Work out the finished part from the listing and answer in its coordinate system (mm). A direction names the side the tool comes from. Give positions to 0.01 mm unless a question says otherwise; leave off trailing zeros. Write each loop counter-clockwise with the first axis right and the second up, starting at its lowest first coordinate (ties: lowest second). Pieces come first, ordered by that corner, then holes. Notation, with made-up numbers: (51, -3) -> (98, -3) arc R32 cw to (98, 26) -> close; hole circle Ø1 at (22, -38). An arc over 180 degrees is marked (long way). Use a Markdown table: item, result. Add a question column.
Q1. Section B-B, the plane z = 45 is taken. Give the vertices of the cut face in (x, y).
Q2. Section A-A, the plane y = -6 is taken. Give the vertices of the cut face in (x, z).
Q3. Section C-C, the plane x = -17 is taken. Give the vertices of the cut face in (y, z).
Q4. For faces 1 (the face through (0, -7, 65)), 2 (the face through (-1, -14, 0.5)), 3 (the face through (3.3, -2.53, -1.23)), determine the directions among +Z, -Z, +X, -X, +Y, -Y from which every point of the face is accessible in a straight line to the end or side of a thin tool.
Q5. Each of these flat-tipped pins is pushed along its axis until it touches: pin 1 Ø3 at (y, z) = (-11, 14.5) entering from +X; pin 2 Ø3 at (x, y) = (9.5, 5.5) entering from -Z; pin 3 Ø4 at (x, z) = (-18, 30) entering from -Y. Where does it stop, or does it pass through?
Q6. Section D-D, the plane y = 6.5 is taken. Give the vertices of the cut face in (x, z).
Q7. Consider line 1 (Z direction, x = 14.5, y = 13.5); line 2 (Y direction, x = 0, z = 66.4); line 3 (X direction, y = 5.5, z = 54.5). Determine where each line is inside the solid, lowest interval first.
Q8. For a pull along Z with two mould halves and no side action, classify faces 4 (the face through (7.31, 12.62, 55.27)), 5 (the face through (-31.096, 0.559, 32.99)), 6 (the face through (6.68, 12.64, 11.65)), 7 (the face through (0, 0, 2.5)) as pulls with the +Z half, pulls with the -Z half, needs draft (parallel to the pull), parting line crosses it, or undercut.
from build123d import *

# Parameters (mm, degrees)
SKETCH_1_R          = 9.1
EXTRUDE_1_DEPTH     = 65
EXTRUDE_2_DEPTH     = 2.5
EXTRUDE_3_DEPTH     = 2.5
SKETCH_7_W          = 30
SKETCH_7_H          = 64
CUT_EXTRUDE_4_DEPTH = 4.5
SKETCH_8_W          = 30
SKETCH_8_H          = 64
CUT_EXTRUDE_5_DEPTH = 4.5
SKETCH_4_R          = 4.159545235
SKETCH_4_R_2        = 2.25
EXTRUDE_4_DEPTH     = 2.5
SKETCH_10_R         = 2.25
CUT_EXTRUDE_6_DEPTH = 2.5
SKETCH_11_R         = 4.25
SKETCH_11_R_2       = 2.25
EXTRUDE_5_DEPTH     = 4.5
SKETCH_3_R          = 4.25
SKETCH_3_R_2        = 2.25
EXTRUDE_6_DEPTH     = 2.5


with BuildPart() as part:
    # Эскиз1 → Бобышка-Вытянуть1 (new body)
    with BuildSketch(Plane.XY):
        with BuildLine():
            Line((-15.348477888, 15.359663741), (14.645527362, 14.759956259))
            ThreePointArc((14.645527362, 14.759956259), (29.785323334, -0.997609119), (14.027757956, -16.137405091))
            Line((14.027757956, -16.137405091), (-15.966247294, -15.537697609))
            ThreePointArc((-15.966247294, -15.537697609), (-31.106043266, 0.219867769), (-15.348477888, 15.359663741))
        make_face()
        with Locations((-15.657362591, -0.089016934)):
            Circle(SKETCH_1_R, mode=Mode.SUBTRACT)
        with Locations((14.336642659, -0.688724416)):
            Circle(SKETCH_1_R, mode=Mode.SUBTRACT)
    extrude(amount=EXTRUDE_1_DEPTH)

    # Эскиз2 → Бобышка-Вытянуть2 (add)
    with BuildSketch(Plane.XY.offset(65)):
        with BuildLine():
            Line((-15.966247294, -15.537697609), (14.027757956, -16.137405091))
            ThreePointArc((14.027757956, -16.137405091), (29.785323334, -0.997609119), (14.645527362, 14.759956259))
            Line((14.645527362, 14.759956259), (-15.348477888, 15.359663741))
            ThreePointArc((-15.348477888, 15.359663741), (-31.106043266, 0.219867769), (-15.966247294, -15.537697609))
        make_face()
        with BuildLine():
            Line((-15.378463262, 13.859963479), (14.615541988, 13.260255996))
            ThreePointArc((14.615541988, 13.260255996), (28.285623072, -0.967623745), (14.05774333, -14.637704829))
            Line((14.05774333, -14.637704829), (-15.93626192, -14.037997346))
            ThreePointArc((-15.93626192, -14.037997346), (-29.606343003, 0.189882395), (-15.378463262, 13.859963479))
        make_face(mode=Mode.SUBTRACT)
    extrude(amount=EXTRUDE_2_DEPTH)

    # Эскиз5 → Бобышка-Вытянуть3 (add)
    with BuildSketch(Plane(origin=(0, 0, 0), x_dir=(-1, 0, 0), z_dir=(0, 0, -1))):
        with BuildLine():
            Line((15.966247294, -15.537697609), (-14.027757956, -16.137405091))
            ThreePointArc((-14.027757956, -16.137405091), (-29.785323334, -0.997609119), (-14.645527362, 14.759956259))
            Line((-14.645527362, 14.759956259), (15.348477888, 15.359663741))
            ThreePointArc((15.348477888, 15.359663741), (31.106043266, 0.219867769), (15.966247294, -15.537697609))
        make_face()
        with BuildLine():
            Line((-14.615541988, 13.260255996), (15.378463262, 13.859963479))
            ThreePointArc((15.378463262, 13.859963479), (29.606343003, 0.189882395), (15.93626192, -14.037997346))
            Line((15.93626192, -14.037997346), (-14.05774333, -14.637704829))
            ThreePointArc((-14.05774333, -14.637704829), (-28.285623072, -0.967623745), (-14.615541988, 13.260255996))
        make_face(mode=Mode.SUBTRACT)
    extrude(amount=EXTRUDE_3_DEPTH)

    # Эскиз7 → Вырез-Вытянуть4 (cut)
    with BuildSketch(Plane(origin=(0.300848748, 15.046767274, 0), x_dir=(0.999800175, -0.019990249, 0), z_dir=(0.019990249, 0.999800175, 0))):
        with Locations((-0.652454388, -32.5)):
            Rectangle(SKETCH_7_W, SKETCH_7_H)
    extrude(amount=-CUT_EXTRUDE_4_DEPTH, mode=Mode.SUBTRACT)

    # Эскиз8 → Вырез-Вытянуть5 (cut)
    with BuildSketch(Plane(origin=(-0.316920658, -15.850594076, 0), x_dir=(-0.999800175, 0.019990249, 0), z_dir=(-0.019990249, -0.999800175, 0))):
        with Locations((0.652454388, -32.5)):
            Rectangle(SKETCH_8_W, SKETCH_8_H)
    extrude(amount=-CUT_EXTRUDE_5_DEPTH, mode=Mode.SUBTRACT)

    # Эскиз4 → Бобышка-Вытянуть4 (add)
    with BuildSketch(Plane(origin=(0, 0, 0), x_dir=(-1, 0, 0), z_dir=(0, 0, -1))):
        Circle(SKETCH_4_R)
        Circle(SKETCH_4_R_2, mode=Mode.SUBTRACT)
    extrude(amount=EXTRUDE_4_DEPTH)

    # Эскиз10 → Вырез-Вытянуть6 (cut)
    with BuildSketch(Plane(origin=(0, 0, 0), x_dir=(-1, 0, 0), z_dir=(0, 0, -1))):
        Circle(SKETCH_10_R)
    extrude(amount=-CUT_EXTRUDE_6_DEPTH, mode=Mode.SUBTRACT)

    # Эскиз11 → Бобышка-Вытянуть5 (add)
    with BuildSketch(Plane(origin=(0.210892625, 10.547666486, 0), x_dir=(0.999800175, -0.019990249, 0), z_dir=(0.019990249, 0.999800175, 0))):
        with Locations((7.347545612, -7.5)):
            Circle(SKETCH_11_R)
        with Locations((7.347545612, -7.5)):
            Circle(SKETCH_11_R_2, mode=Mode.SUBTRACT)
        with Locations((-8.652454388, -7.5)):
            Circle(SKETCH_11_R)
        with Locations((-8.652454388, -7.5)):
            Circle(SKETCH_11_R_2, mode=Mode.SUBTRACT)
        with Locations((7.347545612, -57.5)):
            Circle(SKETCH_11_R)
        with Locations((7.347545612, -57.5)):
            Circle(SKETCH_11_R_2, mode=Mode.SUBTRACT)
        with Locations((-8.652454388, -57.5)):
            Circle(SKETCH_11_R)
        with Locations((-8.652454388, -57.5)):
            Circle(SKETCH_11_R_2, mode=Mode.SUBTRACT)
    extrude(amount=EXTRUDE_5_DEPTH)

    # Эскиз3 → Бобышка-Вытянуть6 (add)
    with BuildSketch(Plane.XY.offset(65)):
        Circle(SKETCH_3_R)
        Circle(SKETCH_3_R_2, mode=Mode.SUBTRACT)
    extrude(amount=EXTRUDE_6_DEPTH)


solid = part.part
Result set:
| question | item | result |
|---|---|---|
| 1 | outline | (-15.97, -15.54) -> (-15.88, -11.04) -> (14.12, -11.64) -> (14.03, -16.14) arc R15.45 ccw to (14.65, 14.76) -> (14.56, 10.26) -> (-15.44, 10.86) -> (-15.35, 15.36) arc R15.45 ccw to start; hole circle Ø18.2 at (-15.66, -0.09); hole circle Ø18.2 at (14.34, -0.69) |
| 2 | outline | (-29.93, -2.5) -> (-28.3, -2.5) -> (-28.3, 0) -> (-22.58, 0) -> (-22.58, 65) -> (-28.3, 65) -> (-28.3, 67.5) -> (-29.93, 67.5) -> close; (-8.74, 0) -> (6.95, 0) -> (6.95, 65) -> (-8.74, 65) -> close; (21.73, 0) -> (27.24, 0) -> (27.24, -2.5) -> (28.85, -2.5) -> (28.85, 67.5) -> (27.24, 67.5) -> (27.24, 65) -> (21.73, 65) -> close |
| 3 | outline | (-15.48, -2.5) -> (-13.98, -2.5) -> (-13.98, 0) -> (-9.09, 0) -> (-9.09, 65) -> (-13.98, 65) -> (-13.98, 67.5) -> (-15.48, 67.5) -> close; (8.91, 0) -> (13.8, 0) -> (13.8, -2.5) -> (15.3, -2.5) -> (15.3, 67.5) -> (13.8, 67.5) -> (13.8, 65) -> (8.91, 65) -> close |
| 4 | face 1 | +Z |
| 4 | face 2 | -Y |
| 4 | face 3 | -Z |
| 5 | pin 1 | stops at x = 27.03 |
| 5 | pin 2 | stops at z = 0 |
| 5 | pin 3 | stops at y = -15.54 |
| 6 | outline | (-29.63, -2.5) -> (-27.96, -2.5) -> (-27.96, 0) -> (-21.93, 0) -> (-21.93, 65) -> (-27.96, 65) -> (-27.96, 67.5) -> (-29.63, 67.5) -> close; (-9.38, 0) -> (8.76, 0) -> (8.76, 65) -> (-9.38, 65) -> close; (19.92, 0) -> (26.29, 0) -> (26.29, -2.5) -> (28.01, -2.5) -> (28.01, 67.5) -> (26.29, 67.5) -> (26.29, 65) -> (19.92, 65) -> close |
| 7 | line 1 | z = -2.5 to 0.5, 64.5 to 67.5 |
| 7 | line 2 | y = -15.86 to -14.36, -4.25 to -2.25, 2.25 to 4.25, 13.55 to 15.05 |
| 7 | line 3 | x = -30.06 to -22.84, -8.48 to 7.67, 21.01 to 28.49 |
| 8 | face 4 | undercut |
| 8 | face 5 | needs draft |
| 8 | face 6 | undercut |
| 8 | face 7 | pulls with the -Z half |
